```python
from build123d import *

# Parameters (mm, degrees)
SKETCH1_W           = 175
SKETCH1_H           = 175
BOSS_EXTRUDE1_DEPTH = 1
SKETCH2_W           = 1.2
SKETCH2_H           = 175
BOSS_EXTRUDE2_DEPTH = 250
SKETCH3_W           = 80
SKETCH3_H           = 175
BOSS_EXTRUDE3_DEPTH = 1
SKETCH4_R           = 2.5
CUT_EXTRUDE1_DEPTH  = 10
SKETCH6_R           = 2.5
CUT_EXTRUDE2_DEPTH  = 300


with BuildPart() as part:
    # Sketch1 → Boss-Extrude1 (new body)
    with BuildSketch(Plane(origin=(0, 0, 0), x_dir=(1, 0, 0), z_dir=(0, 1, 0))):
        Rectangle(SKETCH1_W, SKETCH1_H)
    extrude(amount=BOSS_EXTRUDE1_DEPTH)

    # Sketch2 → Boss-Extrude2 (add)
    with BuildSketch(Plane.XZ):
        with Locations((-88.1, 0)):
            Rectangle(SKETCH2_W, SKETCH2_H)
        with Locations((88.1, 0)):
            Rectangle(SKETCH2_W, SKETCH2_H)
    extrude(amount=-BOSS_EXTRUDE2_DEPTH)

    # Sketch3 → Boss-Extrude3 (add)
    with BuildSketch(Plane(origin=(0, 250, 0), x_dir=(1, 0, 0), z_dir=(0, 1, 0))):
        with Locations((-127.5, 0)):
            Rectangle(SKETCH3_W, SKETCH3_H)
        with Locations((127.5, 0)):
            Rectangle(SKETCH3_W, SKETCH3_H)
    extrude(amount=BOSS_EXTRUDE3_DEPTH)

    # Sketch4 → Cut-Extrude1 (cut)
    with BuildSketch(Plane(origin=(0, 251, 0), x_dir=(1, 0, 0), z_dir=(0, 1, 0))):
        with Locations(Location((131.5, 19.6, 0), (0, 0, 270))):
            Circle(SKETCH4_R)
        with Locations(Location((131.5, -19.6, 0), (0, 0, 90))):
            Circle(SKETCH4_R)
        with Locations(Location((-131.5, -19.6, 0), (0, 0, 270))):
            Circle(SKETCH4_R)
        with Locations(Location((-131.5, 19.6, 0), (0, 0, 90))):
            Circle(SKETCH4_R)
    extrude(amount=-CUT_EXTRUDE1_DEPTH, mode=Mode.SUBTRACT)

    # Sketch6 → Cut-Extrude2 (cut)
    with BuildSketch(Plane(origin=(88.7, 0, 0), x_dir=(0, 0, -1), z_dir=(1, 0, 0))):
        with Locations((70.077336333, 25)):
            Circle(SKETCH6_R)
        with Locations((70.077336333, 75)):
            Circle(SKETCH6_R)
        with Locations((70.077336333, 125)):
            Circle(SKETCH6_R)
        with Locations(Location((-70.077336333, 125, 0), (0, 0, 180))):
            Circle(SKETCH6_R)
        with Locations(Location((-70.077336333, 75, 0), (0, 0, 180))):
            Circle(SKETCH6_R)
        with Locations(Location((-70.077336333, 25, 0), (0, 0, 180))):
            Circle(SKETCH6_R)
    extrude(amount=-CUT_EXTRUDE2_DEPTH, mode=Mode.SUBTRACT)


solid = part.part
```
Design review of the part built by this model. Coordinates are the model's own, in mm. A direction names the side the tool comes from. Give positions to 0.01 mm unless a question says otherwise; leave off trailing zeros. Loops run counter-clockwise (first coordinate to the right, second up) from the corner with the lowest first, then second, coordinate; pieces in that order, holes last. Notation, with made-up numbers: (47.5, 17) -> (88.5, 17) arc R31 cw to (88.5, 45) -> close; hole circle Ø7 at (4.25, 64.25). An arc over 180 degrees is marked (long way). Write each question's results on one line, items separated by ' | '.
Q1. Take a section at C-C, the plane x = 63. Write out the cut boundary in (y, z), plus the area to 3 significant figures.
Reply:
outline: (0, -87.5) -> (1, -87.5) -> (1, 87.5) -> (0, 87.5) -> close | area: 175 mm²
Q2. Machinability: for faces 4 (the face through (-1, 0, 1)), 5 (the face through (128, 250, -1)), 6 (the face through (87.5, 124, -1)), which of the approach directions +Z, -Z, +X, -X, +Y, -Y give a long, thin tool a straight path to every point of the face, cutting with its end or side? Answer none if there is none.
Reply:
face 4: +Z, -Z, +X, -X, -Y | face 5: +Z, -Z, +X, -Y | face 6: +Z, -Z, +Y
Q3. Take a section at B-B, the plane z = 44. Write out the cut boundary in (x, y), plus the area to 3 significant figures.
Reply:
outline: (-167.5, 250) -> (-88.7, 250) -> (-88.7, 0) -> (88.7, 0) -> (88.7, 250) -> (167.5, 250) -> (167.5, 251) -> (87.5, 251) -> (87.5, 1) -> (-87.5, 1) -> (-87.5, 251) -> (-167.5, 251) -> close | area: 935 mm²
Q4. Wall thickness on L1, parallel to X at y = 74, z = -14.5; L2, parallel to Y at x = 94, z = -48.5; L3, parallel to Y at x = -46.5, z = -28.5: over which ranges is each line inside the solid? List them lowest first.
Reply:
L1: x = -88.7 to -87.5, 87.5 to 88.7 | L2: y = 250 to 251 | L3: y = 0 to 1
Q5. The part is to be moulded in two halves that separate along X. For faces 1 (the face through (-129, 250, -1)), 2 (the face through (-88.7, 123, -1)), 3 (the face through (-1, 1, -1)), say which applies: +X half, -X half, draft (parallel to the pull), parting line (faces both ways), or undercut.
Reply:
face 1: draft | face 2: -X half | face 3: undercut
Q6. Take a section at A-A, the plane y = 175. Write out the cut boundary in (x, z), plus the area to 3 significant figures.
Reply:
outline: (-88.7, -87.5) -> (-87.5, -87.5) -> (-87.5, 87.5) -> (-88.7, 87.5) -> close; (87.5, -87.5) -> (88.7, -87.5) -> (88.7, 87.5) -> (87.5, 87.5) -> close | area: 420 mm²
Q7. For pin 1 Ø12 at (y, z) = (27.5, 14) entering from -X; pin 2 Ø1.5 at (x, z) = (-30.5, 1) entering from -Y; pin 3 Ø6 at (y, z) = (91, 69.5) entering from +X, all flat-tipped, find the tip position at first contact; note any pin that passes through.
Reply:
pin 1: stops at x = -88.7 | pin 2: stops at y = 0 | pin 3: stops at x = 88.7
